```python
from build123d import *

# Parameters (mm, degrees)
SKETCH1_W                 = 8.5
SKETCH1_H                 = 15
BOSS_EXTRUDE1_DEPTH       = 4.65
F_3_0MM_DOWEL_HOLE1_D     = 3
F_3_0MM_DOWEL_HOLE1_DEPTH = 5
F_3_0MM_DOWEL_HOLE1_TIP   = 0.901290929
SKETCH2_R                 = 2.85
CUT_EXTRUDE2_DEPTH        = 2.2


with BuildPart() as part:
    # Sketch1 → Boss-Extrude1 (new body)
    with BuildSketch(Plane.XY):
        Rectangle(SKETCH1_W, SKETCH1_H)
    extrude(amount=BOSS_EXTRUDE1_DEPTH)

    # Ø3.0mm Dowel Hole1
    with Locations(Plane.XY.offset(4.65)):
        with Locations((0, 4.175), (0, -4.175)):
            Hole(F_3_0MM_DOWEL_HOLE1_D / 2, depth=F_3_0MM_DOWEL_HOLE1_DEPTH)
            with Locations((0, 0, -(F_3_0MM_DOWEL_HOLE1_DEPTH + F_3_0MM_DOWEL_HOLE1_TIP / 2))):  # 118° drill point
                Cone(0, F_3_0MM_DOWEL_HOLE1_D / 2, F_3_0MM_DOWEL_HOLE1_TIP, mode=Mode.SUBTRACT)

    # Sketch2 → Cut-Extrude2 (cut)
    with BuildSketch(Plane.XY.offset(4.65)):
        with Locations((0, -4.175)):
            Circle(SKETCH2_R)
        with Locations((0, 4.175)):
            Circle(SKETCH2_R)
    extrude(amount=-CUT_EXTRUDE2_DEPTH, mode=Mode.SUBTRACT)


solid = part.part
```
The listing builds one solid part. Answer for the finished solid, in the listing's coordinates (mm). A direction names the side the tool comes from. Give positions to 0.01 mm unless a question says otherwise; leave off trailing zeros. Order: outer loops, then holes, each group sorted by start corner. A loop starts at its lowest first (then second) coordinate and runs counter-clockwise, first axis right, second up. Notation, with made-up numbers: (-20.75, -15) -> (25.25, -15) arc R13 ccw to (25.25, 4) -> close; hole circle Ø9 at (70, 35). An arc over 180 degrees is marked (long way). Answer as CSV lines item,"result". Start each with the question number.
Q1. Find the intervals of material crossed by L1, parallel to Y at x = 0, z = 0.8 (3 decimals); L2, parallel to Y at x = 0, z = 2.95 (3 decimals); L3, parallel to Z at x = 1.75, y = -3.5, in increasing order.
Q2. A cutting plane is placed at B-B (y = 5.25). Determine the outline of the cut face in (x, z).
Q3. A cutting plane is placed at C-C (z = 0.4). Determine the outline of the cut face in (x, y) (3 decimals).
Q4. A cutting plane is placed at A-A (x = 0). Determine the outline of the cut face in (y, z) (3 decimals).
Q5. Given pin 1 (1 mm diameter, centred on x = 0, y = 1, fed in from -Z); pin 2 (1.7 mm diameter, centred on x = 1, y = 5, fed in from +Z); pin 3 (1.8 mm diameter, centred on x = 0, y = -4.175, fed in from -Z), each flat-ended and moving along its own axis, determine where each tip first touches the part or whether it passes through.
Q6. Determine the mould class of faces 1 (the flat face through (0, 7.5, 2)), 2 (the flat face through (0, 0, 0)), 3 (the flat face through (1.2, -5.4, 2.45)) for opening direction Y: pulls with the +Y half, pulls with the -Y half, needs draft (parallel to the pull), parting line crosses it, or undercut.
Q7. Which of the six approach directions +Z, -Z, +X, -X, +Y, -Y give full straight-line access (tool end or side, diameter ignored) to faces 4 (the cylindrical face through (0.2, -2.69, 1.21)), 5 (the cylindrical face through (-0.618, -6.957, 3.565))?
Q8. A cutting plane is placed at D-D (x = -1.75). Determine the outline of the cut face in (y, z).
Results found:
1,L1,"-7.5 to -5.675, -2.675 to 2.675, 5.675 to 7.5"
1,L2,"-7.5 to -7.025, -1.325 to 1.325, 7.025 to 7.5"
1,L3,"0 to 2.45"
2,outline,"(-4.25, 0) -> (-1.05, 0) -> (-1.05, 2.45) -> (-2.64, 2.45) -> (-2.64, 4.65) -> (-4.25, 4.65) -> close; (1.05, 0) -> (4.25, 0) -> (4.25, 4.65) -> (2.64, 4.65) -> (2.64, 2.45) -> (1.05, 2.45) -> close"
3,outline,"(-4.25, -7.5) -> (4.25, -7.5) -> (4.25, 7.5) -> (-4.25, 7.5) -> close; hole circle Ø3 at (0, -4.175); hole circle Ø3 at (0, 4.175)"
4,outline,"(-7.5, 0) -> (-5.675, 0) -> (-5.675, 2.45) -> (-7.025, 2.45) -> (-7.025, 4.65) -> (-7.5, 4.65) -> close; (-2.675, 0) -> (2.675, 0) -> (2.675, 2.45) -> (1.325, 2.45) -> (1.325, 4.65) -> (-1.325, 4.65) -> (-1.325, 2.45) -> (-2.675, 2.45) -> close; (5.675, 0) -> (7.5, 0) -> (7.5, 4.65) -> (7.025, 4.65) -> (7.025, 2.45) -> (5.675, 2.45) -> close"
5,pin 1,"z = 0"
5,pin 2,"z = 2.45"
5,pin 3,"through"
6,face 1,"pulls with the +Y half"
6,face 2,"needs draft"
6,face 3,"undercut"
7,face 4,"+Z, -Z"
7,face 5,"+Z"
8,outline,"(-7.5, 0) -> (7.5, 0) -> (7.5, 4.65) -> (6.42, 4.65) -> (6.42, 2.45) -> (1.93, 2.45) -> (1.93, 4.65) -> (-1.93, 4.65) -> (-1.93, 2.45) -> (-6.42, 2.45) -> (-6.42, 4.65) -> (-7.5, 4.65) -> close"
